Model file for the job. Use its own axes, mm. Give positions to 0.01 mm unless a question says otherwise; leave off trailing zeros. Order: outer loops, then holes, each group sorted by start corner. A loop starts at its lowest first (then second) coordinate and runs counter-clockwise, first axis right, second up. Notation, with made-up numbers: M 14,0.25 L 35,0.25 A17 cw 35,8.25 Z; hole C -16,62 d4. An arc over 180 degrees is marked long. Return JSON: item names as keys, results as strings. Group by question number.
1. Slice it at C-C on y = -0.4. List the corners of the cut face in (x, z), then the cut area to 3 significant figures.
2. Slice it at B-B on x = 18.5. List the corners of the cut face in (y, z).
3. Wall check: probe 1 along Z at (x, y) = (10.5, -0.5); probe 2 along X at (y, z) = (-0.9, -15); probe 3 along Z at (x, y) = (16.75, 0.7). Give the ranges that are in metal, low to high. Write a range as [from, to].
4. Slice it at A-A on z = -37.5. List the corners of the cut face in (x, y).
5. Pin check, flat tips, straight feed: pin 1 (8 mm diameter, centred on x = 8, z = -9, fed in from -Y); pin 2 (1 mm diameter, centred on x = 3.5, y = 0, fed in from -Z); pin 3 (5 mm diameter, centred on x = 3.5, z = -54, fed in from -Y). Stop position of each tip, or through.
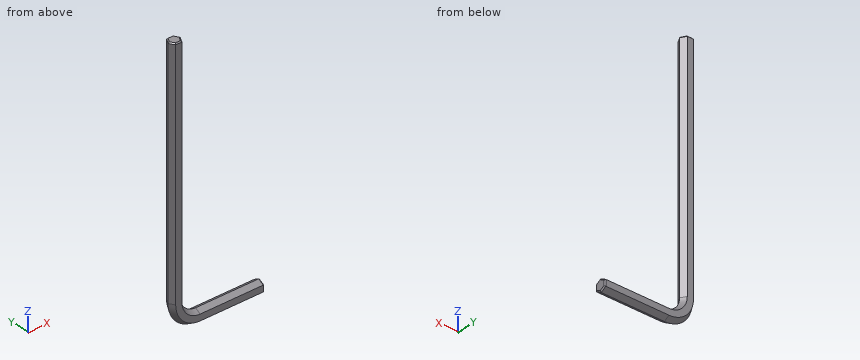
from build123d import *

# Parameters (mm, degrees)
CHAMFER1_SIZE = 0.25
CHAMFER2_SIZE = 0.25


with BuildPart() as part:
    # Sweep1: sweep along a path in Sketch2
    with BuildLine(Plane(origin=(0, 0, 0), x_dir=(1, 0, 0), z_dir=(0, 1, 0))) as sweep1_path:
        Line((0, 0), (0, 55))
        ThreePointArc((0, 55), (1.464466094, 58.535533906), (5, 60))
        Line((5, 60), (20, 60))
    # Sketch1 → Sweep1 (sweep)
    with BuildSketch(Plane.XY):
        Polygon((0.721687836, 1.25), (-0.721687836, 1.25), (-1.443375673, 0), (-0.721687836, -1.25), (0.721687836, -1.25), (1.443375673, 0), align=None)
    sweep(path=sweep1_path.line)

    # Chamfer1
    chamfer1_edges = [part.edges().sort_by_distance(p)[0] for p in [
        (20, -1.25, -60),
        (20, -0.625, -58.917468245),
        (20, 0.625, -58.917468245),
        (20, 1.25, -60),
        (20, 0.625, -61.082531755),
        (20, -0.625, -61.082531755),
    ]]
    chamfer(chamfer1_edges, length=CHAMFER1_SIZE)

    # Chamfer2
    chamfer2_edges = [part.edges().sort_by_distance(p)[0] for p in [
        (0, 1.25, 0),
        (-1.082531755, 0.625, 0),
        (-1.082531755, -0.625, 0),
        (0, -1.25, 0),
        (1.082531755, -0.625, 0),
        (1.082531755, 0.625, 0),
    ]]
    chamfer(chamfer2_edges, length=CHAMFER2_SIZE)


solid = part.part
Result:
{
 "1": {"outline": "M -1.21,-55 A6.21 ccw 5,-61.21 L 19.75,-61.21 L 20,-60.92 L 20,-59.08 L 19.75,-58.79 L 5,-58.79 A3.79 cw 1.21,-55 L 1.21,-0.25 L 0.92,0 L -0.92,0 L -1.21,-0.25 Z", "area": "189 mm2"},
 "2": {"outline": "M -1.25,-60.72 L 0,-61.44 L 1.25,-60.72 L 1.25,-59.28 L 0,-58.56 L -1.25,-59.28 Z"},
 "3": {"probe 1": "z = [-61.15, -58.85]", "probe 2": "x = [-0.92, 0.92]", "probe 3": "z = [-61.04, -58.96]"},
 "4": {"outline": "M -1.44,0 L -0.72,-1.25 L 0.72,-1.25 L 1.44,0 L 0.72,1.25 L -0.72,1.25 Z"},
 "5": {"pin 1": "passes through", "pin 2": "stops at z = -61.37", "pin 3": "stops at y = -0.77"}
}
